Answer from the drawing. Dimensions are ordinates in mm from the lowest x, y and z of the part. Coordinates: 2 decimals unless noted, no trailing zeros. Loops run counter-clockwise (first coordinate to the right, second up) from the corner with the lowest first, then second, coordinate; pieces in that order, holes last. Notation, with made-up numbers: (24.5, 26.25) -> (36.5, 26.25) arc R16 cw to (36.5, 50.25) -> close; hole circle Ø2 at (53, 50). An arc over 180 degrees is marked (long way). Use a Markdown table: item, result.
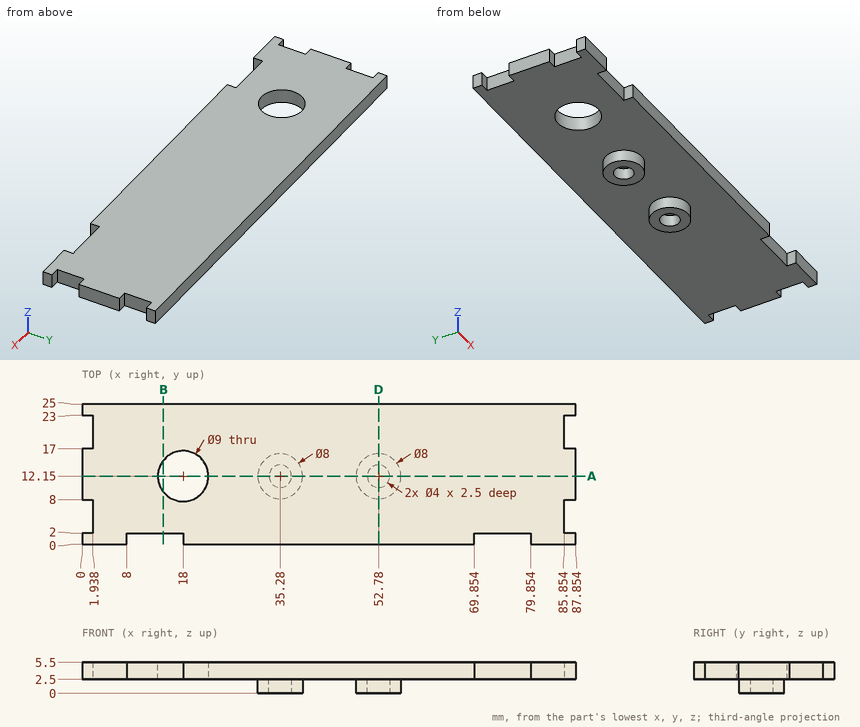
Q1. Given pin 1 Ø1.6 at (x, z) = (87, 4.5) entering from -Y; pin 2 Ø2.5 at (y, z) = (20, 4.5) entering from -X; pin 3 Ø3.5 at (x, y) = (52.78, 12.15) entering from -Z; pin 4 Ø1.5 at (x, z) = (10.5, 4) entering from -Y, each flat-ended and moving along its own axis, determine where each tip first touches the part or whether it passes through.
Solved:
| item | result |
|---|---|
| pin 1 | y = 0 |
| pin 2 | x = 1.94 |
| pin 3 | z = 2.5 |
| pin 4 | y = 2 |
Q2. Consider line 1 (Y direction, x = 35.28, z = 1.55); line 2 (Z direction, x = 23, y = 15); line 3 (Y direction, x = 72.5, z = 3.65). Determine where each line is inside the solid, lowest interval first. Write a range as [from, to].
Solved:
| item | result |
|---|---|
| line 1 | [8.15, 10.15], [14.15, 16.15] |
| line 2 | [2.5, 5.5] |
| line 3 | [2, 25] |
Q3. Section A-A on y = 12.15 is taken. Determine the outline of the cut face in (x, z) (1 decimal).
Solved:
| item | result |
|---|---|
| outline | (0, 2.5) -> (13.5, 2.5) -> (13.5, 5.5) -> (0, 5.5) -> close; (22.5, 2.5) -> (31.3, 2.5) -> (31.3, 0) -> (33.3, 0) -> (33.3, 2.5) -> (37.3, 2.5) -> (37.3, 0) -> (39.3, 0) -> (39.3, 2.5) -> (48.8, 2.5) -> (48.8, 0) -> (50.8, 0) -> (50.8, 2.5) -> (54.8, 2.5) -> (54.8, 0) -> (56.8, 0) -> (56.8, 2.5) -> (87.9, 2.5) -> (87.9, 5.5) -> (22.5, 5.5) -> close |
Q4. Section D-D on x = 52.78 is taken. Determine the outline of the cut face in (y, z).
Solved:
| item | result |
|---|---|
| outline | (0, 2.5) -> (8.15, 2.5) -> (8.15, 0) -> (10.15, 0) -> (10.15, 2.5) -> (14.15, 2.5) -> (14.15, 0) -> (16.15, 0) -> (16.15, 2.5) -> (25, 2.5) -> (25, 5.5) -> (0, 5.5) -> close |
Q5. Section B-B on x = 14.5 is taken. Determine the outline of the cut face in (y, z).
Solved:
| item | result |
|---|---|
| outline | (2, 2.5) -> (9.32, 2.5) -> (9.32, 5.5) -> (2, 5.5) -> close; (14.98, 2.5) -> (25, 2.5) -> (25, 5.5) -> (14.98, 5.5) -> close |
